Build history of the part. All positions in model axes, mm. A direction names the side the tool comes from. Round coordinates to 2 decimals unless told otherwise and drop trailing zeros. Order: outer loops, then holes, each group sorted by start corner. A loop starts at its lowest first (then second) coordinate and runs counter-clockwise, first axis right, second up. Notation, with made-up numbers: M 40,32 L 79,32 A11 cw 79,43 Z; hole C 34,-33 d5. An arc over 180 degrees is marked long. One line per item, written item: value. Start each with the question number.
Item 1: Pin check, flat tip, straight feed: pin 1 (0.8 mm diameter, centred on y = -19.5, z = 0.5, fed in from -X). Stop position of the tip, or through.
Item 2: Band-saw the part on A-A, the plane x = 13. Write the cut outline in (y, z).
Item 3: Tool access for faces 5 (the flat face through (26.673, 44.293, 0.74)), 6 (the flat face through (9.6, 21.1, 0)): list every direction of +Z, -Z, +X, -X, +Y, -Y with a clear straight run to the whole face (end or side of a thin tool).
Item 4: Probe L1, parallel to Y at x = 42, z = 1.1; L2, parallel to Y at x = 36.5, z = 0.9; L3, parallel to X at y = -11.5, z = 1.05. List the from-to ranges inside material, lowest first.
Item 5: Band-saw the part on C-C, the plane y = -32.5. Write the cut outline in (x, z).
Item 6: Two-plate mould, pull along Y, no slides. Class faces 1 (the flat face through (30, -30, 1)), 2 (the flat face through (35.35, 49.3, 0.74)), 3 (the flat face through (9.6, 21.1, 1.5)), 4 (the flat face through (37.25, -23.11, 0.74)): +Y half, -Y half, draft (parallel to the pull), parting line (faces both ways), or undercut.
Item 7: Band-saw the part on B-B, the plane z = 1.15. Write the cut outline in (x, y), then the cut area to 3 significant figures.
Item 8: Band-saw the part on D-D, the plane x = 35. Write the cut outline in (y, z).
```python
from build123d import *

# Parameters (mm, degrees)
F1_DEPTH = 1.5


with BuildPart() as f1:
    # F0 (on Top) → F1 (new body)
    with BuildSketch(Plane.XY):
        Polygon((60, 0), (0, 0), (60, -60), align=None)
        Polygon((50, -10), (50, -35.857864), (24.142136, -10), align=None, mode=Mode.SUBTRACT)
        Polygon((0, 100), (0, 0), (60, 0), (10, 100), align=None)
        Polygon((43.81966, 10), (10, 10), (10, 77.63932), align=None, mode=Mode.SUBTRACT)
    extrude(amount=F1_DEPTH)


solid = f1.part
```
Output:
1. pin 1: stops at x = 19.1
2. outline: M -13,0 L 10,0 L 10,1.5 L -13,1.5 Z; M 71.64,0 L 94,0 L 94,1.5 L 71.64,1.5 Z
3. face 5: +Z, -Z
3. face 6: -Z, +X, -X, +Y, -Y
4. L1: y = -42 to -27.86, -10 to 10, 13.64 to 36
4. L2: y = -36.5 to -22.36, -10 to 10, 24.64 to 47
4. L3: x = 11.5 to 25.64, 50 to 60
5. outline: M 32.5,0 L 46.64,0 L 46.64,1.5 L 32.5,1.5 Z; M 50,0 L 60,0 L 60,1.5 L 50,1.5 Z
6. face 1: -Y half
6. face 2: +Y half
6. face 3: draft
6. face 4: undercut
7. outline: M 0,0 L 60,-60 L 60,0 L 10,100 L 0,100 Z; hole M 10,10 L 43.82,10 L 10,77.64 Z; hole M 24.14,-10 L 50,-35.86 L 50,-10 Z
7. area: 3,820 mm²
8. outline: M -35,0 L -20.86,0 L -20.86,1.5 L -35,1.5 Z; M -10,0 L 10,0 L 10,1.5 L -10,1.5 Z; M 27.64,0 L 50,0 L 50,1.5 L 27.64,1.5 Z
